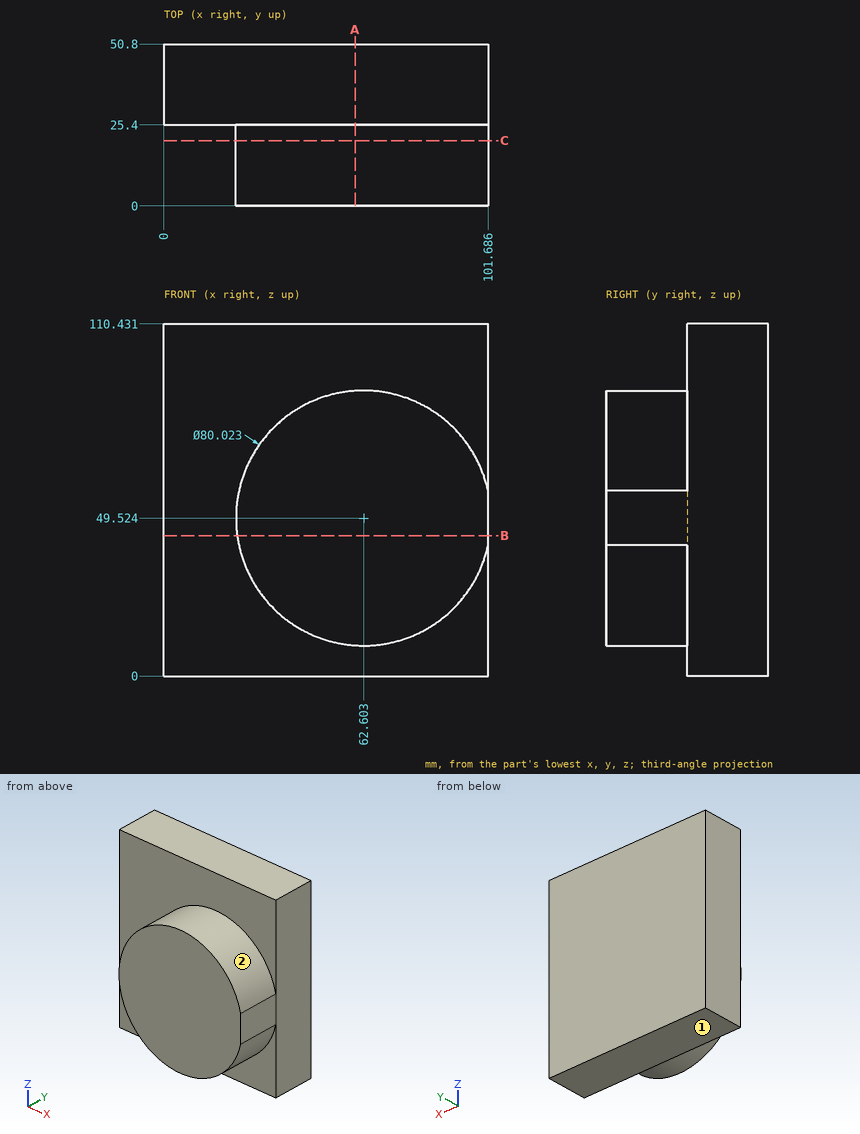
Source: three-view drawing plus pictorial views. Frame: mm from the lowest corner of the part. A direction names the side the tool comes from. Coordinates: 2 decimals unless noted, no trailing zeros. Loops run counter-clockwise (first coordinate to the right, second up) from the corner with the lowest first, then second, coordinate; pieces in that order, holes last. Notation, with made-up numbers: (1, -39.5) - (54, -39.5) arc R36 cw to (54, -1.5) - close; hole circle Ø11 at (7.5, 23.5). An arc over 180 degrees is marked (long way). One line per item, written item: value. Start each with the question number.
1. Ray query, L1, parallel to X at y = 25, z = 48.5 (1 decimal); L2, parallel to Y at x = 11, z = 58; L3, parallel to Z at x = 85, y = 17. Return the intervals inside material, ascending.
2. Section C-C (y = 20.5). Return the cut outline in (x, z) (1 decimal), and give its area (3 significant figures).
3. Section A-A (x = 60). Return the cut outline in (y, z), and give its area (3 significant figures).
4. Section B-B (z = 44). Return the cut outline in (x, y) (1 decimal), and give its area (3 significant figures).
5. Set-up query: the marked faces 1 and 2. Return all of +Z, -Z, +X, -X, +Y, -Y with unobstructed straight access to the full face (end or side cutting, diameter ignored); none if empty.
6. Contact query for flat-ended pins moving along their axis: P1, Ø2, axis at x = 71.5, y = 12, coming from the +Z side; P2, Ø3, axis at y = 10, z = 53.5, coming from the -X side; P3, Ø1.5, axis at x = 91.5, z = 81.5, coming from the -Y side. Output: stop coordinate, or through.
Verdict:
1. L1: x = 22.6 to 101.7
1. L2: y = 25.4 to 50.8
1. L3: z = 16.37 to 82.68
2. outline: (101.7, 41) - (101.7, 58.1) arc R40 ccw (long way) to start
2. area: 5,020 mm2
3. outline: (0, 9.6) - (25.4, 9.6) - (25.4, 0) - (50.8, 0) - (50.8, 110.43) - (25.4, 110.43) - (25.4, 89.45) - (0, 89.45) - close
3. area: 4,830 mm2
4. outline: (0, 25.4) - (23, 25.4) - (23, 0) - (101.7, 0) - (101.7, 50.8) - (0, 50.8) - close
4. area: 4,580 mm2
5. face 1: -Z, +X, -X, +Y, -Y
5. face 2: -Y
6. P1: stops at z = 88.75
6. P2: stops at x = 22.67
6. P3: stops at y = 25.4
